Work out the finished part from the listing and answer in its coordinate system (mm). Face numbers are marked on the shaded views. A direction names the side the tool comes from. Give positions to 0.01 mm unless a question says otherwise; leave off trailing zeros. Loops run counter-clockwise (first coordinate to the right, second up) from the corner with the lowest first, then second, coordinate; pieces in that order, holes last. Notation, with made-up numbers: (-6.75, 15.25) - (3.25, 15.25) arc R25 cw to (3.25, 44.25) - close; hole circle Ø7 at (28.25, 75). An arc over 180 degrees is marked (long way). One line per question, with ' | ' between items. Start each with the question number.
1. Section A-A (y = 0) is taken. Determine the outline of the cut face in (x, z), plus the area to 3 significant figures.
2. Section B-B (z = -8.5) is taken. Determine the outline of the cut face in (x, y).
3. Which of the six approach directions +Z, -Z, +X, -X, +Y, -Y give full straight-line access (tool end or side, diameter ignored) to the marked faces 1 and 2?
4. Section C-C (z = 26) is taken. Determine the outline of the cut face in (x, y), plus the area to 3 significant figures.
5. Find the intervals of material crossed by line 1 (Z direction, x = 1, y = 58); line 2 (X direction, y = -13, z = 10); line 3 (X direction, y = 53, z = -9), in increasing order.
6. Each of these flat-tipped pins is pushed along its axis until it touches: pin 1 (10 mm diameter, centred on x = -16.5, z = -1.5, fed in from -Y); pin 2 (19 mm diameter, centred on x = 17, z = 8, fed in from +Y); pin 3 (1.5 mm diameter, centred on y = 52, z = 11, fed in from -X). Where does it stop, or does it pass through?
7. For a pull along Y with two mould halves and no side action, classify the marked faces 3 and 4 as released by +Y, released by -Y, zero draft, split by the parting line, or undercut.
from build123d import *

# Parameters (mm, degrees)
SKETCH1_R                       = 12.5
BOSS_EXTRUDE1_REACH             = 133.411
SKETCH2_W                       = 160
SKETCH2_H                       = 5
BOSS_EXTRUDE1_DIRECTION_2_REACH = 133.411
SKETCH6_W                       = 17.5
SKETCH6_H                       = 20
BOSS_EXTRUDE2_DEPTH             = 30


with BuildPart() as part:
    # Sketch1 → Revolve1 (revolve)
    with BuildSketch(Plane(origin=(0, 0, 0), x_dir=(1, 0, 0), z_dir=(0, 1, 0))):
        with Locations((80, 0)):
            Circle(SKETCH1_R)
    revolve(axis=Axis((0, 0, 0), (0, 0, -1)))

    # Sketch2 → Boss-Extrude1 (add, up to next)
    with BuildSketch(Plane(origin=(0, 0, 0), x_dir=(1, 0, 0), z_dir=(0, 1, 0)), mode=Mode.PRIVATE) as boss_extrude1_sk1:
        Rectangle(SKETCH2_W, SKETCH2_H)
    boss_extrude1_tool1 = extrude(boss_extrude1_sk1.sketch, amount=BOSS_EXTRUDE1_REACH, mode=Mode.PRIVATE) - part.part
    add(boss_extrude1_tool1.solids().sort_by_distance((0, 0, 0))[0])

    # Sketch2 → Boss-Extrude1 direction 2 (add, up to next)
    with BuildSketch(Plane(origin=(0, 0, 0), x_dir=(1, 0, 0), z_dir=(0, 1, 0)), mode=Mode.PRIVATE) as boss_extrude1_direction_2_sk1:
        Rectangle(SKETCH2_W, SKETCH2_H)
    boss_extrude1_direction_2_tool1 = extrude(boss_extrude1_direction_2_sk1.sketch, amount=-BOSS_EXTRUDE1_DIRECTION_2_REACH, mode=Mode.PRIVATE) - part.part
    add(boss_extrude1_direction_2_tool1.solids().sort_by_distance((0, 0, 0))[0])

    # Sketch4 → Revolve2 (revolve)
    with BuildSketch(Plane(origin=(0, 0, 0), x_dir=(1, 0, 0), z_dir=(0, 1, 0))):
        with BuildLine():
            Line((0, -30), (0, 0))
            Line((0, 0), (10, 0))
            Line((10, 0), (10, -20))
            ThreePointArc((10, -20), (7.071067812, -27.071067812), (0, -30))
        make_face()
    revolve(axis=Axis((0, 0, 30), (0, 0, -1)))

    # Sketch6 → Boss-Extrude2 (add)
    with BuildSketch(Plane(origin=(0, 0, 0), x_dir=(0, 0, -1), z_dir=(1, 0, 0))):
        with Locations((-11.25, 0)):
            Rectangle(SKETCH6_W, SKETCH6_H)
    extrude(amount=BOSS_EXTRUDE2_DEPTH)


solid = part.part
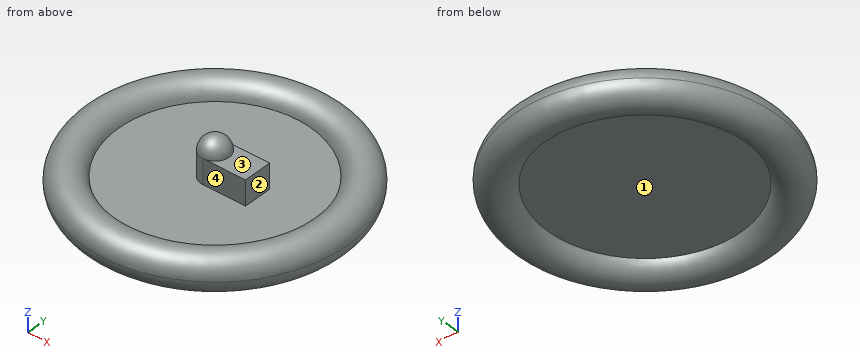
Conclusion:
1) outline: (-67.75, -2.5) - (67.75, -2.5) arc R12.5 ccw (long way) to (67.75, 2.5) - (30, 2.5) - (30, 20) - (10, 20) arc R10 ccw to (-10, 20) - (-10, 2.5) - (-67.75, 2.5) arc R12.5 ccw (long way) to start | area: 2,510 mm²
2) outline: circle Ø178.33 at (0, 0); hole circle Ø141.67 at (0, 0)
3) face 1: -Z | face 2: +Z
4) outline: circle Ø16 at (0, 0) | area: 201 mm²
5) line 1: -2.5 to 2.5 | line 2: -86.53 to -71.32, 71.32 to 86.53 | line 3: -71.09 to -47.73, 47.73 to 71.09
6) pin 1: y = -91.76 | pin 2: y = 91.86 | pin 3: x = -70.05
7) face 3: zero draft | face 4: undercut
